Input: part model. Units: mm. Frame: model coordinates. A direction names the side the tool comes from. Coordinates: 2 decimals unless noted, no trailing zeros. Loops run counter-clockwise (first coordinate to the right, second up) from the corner with the lowest first, then second, coordinate; pieces in that order, holes last. Notation, with made-up numbers: (26.25, 68.5) -> (77.25, 68.5) arc R18 cw to (77.25, 83.5) -> close; hole circle Ø11 at (16.25, 76). An arc over 180 degrees is marked (long way). Answer as a JSON object with one key per item and string values.
from build123d import *

# Parameters (mm, degrees)
Y_KSEKLIK_EKSTR_ZYON1_DEPTH = 30
KES_EKSTR_ZYON2_START       = -22
KES_EKSTR_ZYON2_DEPTH       = 14
IZIM4_R                     = 1.7
KES_EKSTR_ZYON3_DEPTH       = 1.2


with BuildPart() as part:
    # Çizim1 → Yükseklik-Ekstrüzyon1 (new body)
    with BuildSketch(Plane(origin=(0, 0, 0), x_dir=(1, 0, 0), z_dir=(0, 1, 0))):
        with BuildLine():
            Line((0, 0.6), (15, 0.6))
            Line((15, 0.6), (15, -0.6))
            Line((15, -0.6), (0, -0.6))
            ThreePointArc((0, -0.6), (-1.319038138, 4.455873169), (2.301841896, 0.688786378))
            Line((2.301841896, 0.688786378), (1.278801053, 1.315992432))
            ThreePointArc((1.278801053, 1.315992432), (-0.732798966, 3.408818427), (0, 0.6))
        make_face()
    extrude(amount=-Y_KSEKLIK_EKSTR_ZYON1_DEPTH)

    # Çizim3 → Kes-Ekstrüzyon2 (cut)
    with BuildSketch(Plane.XZ.offset(30).offset(KES_EKSTR_ZYON2_START)):
        with BuildLine():
            Line((1.278801053, -1.315992432), (2.301841896, -0.688786378))
            ThreePointArc((2.301841896, -0.688786378), (-1.319038138, -4.455873169), (0, 0.6))
            Line((0, 0.6), (2.7, 0.6))
            Line((2.7, 0.6), (2.7, -0.6))
            Line((2.7, -0.6), (0, -0.6))
            ThreePointArc((0, -0.6), (-0.732798966, -3.408818427), (1.278801053, -1.315992432))
        make_face()
    extrude(amount=KES_EKSTR_ZYON2_DEPTH, mode=Mode.SUBTRACT)

    # Çizim4 → Kes-Ekstrüzyon3 (cut)
    with BuildSketch(Plane(origin=(0, 0, -0.6), x_dir=(-1, 0, 0), z_dir=(0, 0, -1))):
        with Locations((-8, -23)):
            Circle(IZIM4_R)
        with Locations((-8, -7)):
            Circle(IZIM4_R)
    extrude(amount=-KES_EKSTR_ZYON3_DEPTH, mode=Mode.SUBTRACT)


solid = part.part
1. Access query for faces 4 (the face through (4, -30, 0)), 5 (the face through (-1.2, -8, -0.9)), 6 (the face through (1.797, -25.944, -0.998)). Directions: +Z, -Z, +X, -X, +Y, -Y. A direction counts if a zero-diameter tool reaches every point of the face in a straight line with its end or side. Return the directions, or none.
Reply:
{"face 4": "+Z, -Z, +X, -X, -Y", "face 5": "+Z, -Z, -X", "face 6": "+Y, -Y"}
2. Section query C-C (x = 8). Return loops of the section in (y, z), plus the area to 3 significant figures.
Reply:
{"outline": "(-30, -0.6) -> (-24.7, -0.6) -> (-24.7, 0.6) -> (-30, 0.6) -> close; (-21.3, -0.6) -> (-8.7, -0.6) -> (-8.7, 0.6) -> (-21.3, 0.6) -> close; (-5.3, -0.6) -> (0, -0.6) -> (0, 0.6) -> (-5.3, 0.6) -> close", "area": "27.8 mm2"}
3. Mould query, pull axis Y, two halves, no side actions, for faces 1 (the face through (-1.4, -3.94, -4.41)), 2 (the face through (8.37, -8.66, -0.01)), 3 (the face through (4, 0, 0)). Classes: pulls with the +Y half, pulls with the -Y half, needs draft (parallel to the pull), parting line crosses it, or undercut.
Reply:
{"face 1": "needs draft", "face 2": "undercut", "face 3": "pulls with the +Y half"}
4. Pin query (flat end, axial travel): P1, Ø0.6, axis at y = -15, z = 0, coming from the -X side; P2, Ø1.5, axis at x = 5.5, z = -0.5, coming from the +Y side; P3, Ø2, axis at x = 11, y = -9, coming from the -Z side. Return the tip coordinate at first contact, or that it passes through.
Reply:
{"P1": "stops at x = 2.7", "P2": "stops at y = 0", "P3": "stops at z = -0.6"}
5. Section query D-D (y = -27.5). Return loops of the section in (x, z), plus the area to 3 significant figures.
Reply:
{"outline": "(0, -0.6) -> (15, -0.6) -> (15, 0.6) -> (0, 0.6) arc R2.7 ccw (long way) to (2.3, -0.69) -> (1.28, -1.32) arc R1.5 cw (long way) to start", "area": "31.3 mm2"}
6. Section query A-A (z = -2.1). Return loops of the section in (x, y), plus the area to 3 significant figures.
Reply:
{"outline": "(-2.7, -30) -> (-1.5, -30) -> (-1.5, -22) -> (-2.7, -22) -> close; (-2.7, -8) -> (-1.5, -8) -> (-1.5, 0) -> (-2.7, 0) -> close; (1.5, -30) -> (2.7, -30) -> (2.7, -22) -> (1.5, -22) -> close; (1.5, -8) -> (2.7, -8) -> (2.7, 0) -> (1.5, 0) -> close", "area": "38.4 mm2"}
7. Section query B-B (y = -23). Return loops of the section in (x, z).
Reply:
{"outline": "(0, -0.6) -> (6.3, -0.6) -> (6.3, 0.6) -> (0, 0.6) arc R2.7 ccw (long way) to (2.3, -0.69) -> (1.28, -1.32) arc R1.5 cw (long way) to start; (9.7, -0.6) -> (15, -0.6) -> (15, 0.6) -> (9.7, 0.6) -> close"}
8. Line query: line 1 along Y through (x, z) = (8, -0.2); line 2 along X through (y, z) = (-3.5, -2.1); line 3 along Y through (x, z) = (7.5, -0.4). Output: solid intervals per line, ascending.
Reply:
{"line 1": "y = -30 to -24.7, -21.3 to -8.7, -5.3 to 0", "line 2": "x = -2.7 to -1.5, 1.5 to 2.7", "line 3": "y = -30 to -24.62, -21.38 to -8.62, -5.38 to 0"}
